The model under review builds one solid part; all positions refer to its coordinate system, in mm. Face numbers are marked on the shaded views. Round coordinates to 2 decimals unless told otherwise and drop trailing zeros. Order: outer loops, then holes, each group sorted by start corner. A loop starts at its lowest first (then second) coordinate and runs counter-clockwise, first axis right, second up. Notation, with made-up numbers: M 2,7.5 L 56,7.5 A21 ccw 56,27.5 Z; hole C 76,-13.75 d10. An arc over 180 degrees is marked long. Use a Markdown table: item, result. Add a question column.
1. To check wall thickness, follow probe 1 along Y at (x, z) = (0, 87.5); probe 2 along Y at (x, z) = (0, -47); probe 3 along Z at (x, y) = (8.5, -10). State the ranges of each line that lie inside material, in increasing order.
2. Insertion check: P1, Ø15, axis at x = -1, y = -2, coming from the -Z side; P2, Ø2, axis at y = 8, z = 72.5, coming from the +X side; P3, Ø5, axis at x = 8.5, y = 4.5, coming from the -Z side; P4, Ø8, axis at y = 10, z = -82.5, coming from the +X side. Each pin has a flat end and moves straight along its axis. Give the tip position at first contact, or say it passes through.
3. Consider section A-A on x = 0. State the section outline as (y, z) points, then the cut area to 3 significant figures.
4. Consider section C-C on z = 39.5. State the section outline as (x, y) points.
5. The part is to be moulded in two halves that separate along X. For the marked faces 1, 2 and 3, say which applies: +X half, -X half, draft (parallel to the pull), parting line (faces both ways), or undercut.
from build123d import *

# Parameters (mm, degrees)
FILLET1_R = 2


with BuildPart() as part:
    # Sketch1 → Revolve1 (revolve)
    with BuildSketch(Plane.YZ, mode=Mode.PRIVATE) as revolve1_sk:
        Polygon((10, 115), (19, 115), (19, -115), (15, -115), (15, 75), (10, 75), align=None)
    revolve(revolve1_sk.sketch.rotate(Axis((0, 0, 319.317365216), (0, 0, -1)), 90), axis=Axis((0, 0, 319.317365216), (0, 0, -1)))

    # Fillet1
    fillet1_edges = [part.edges().sort_by_distance(p)[0] for p in [
        (-19, 0, 115),
    ]]
    fillet(fillet1_edges, radius=FILLET1_R)


solid = part.part
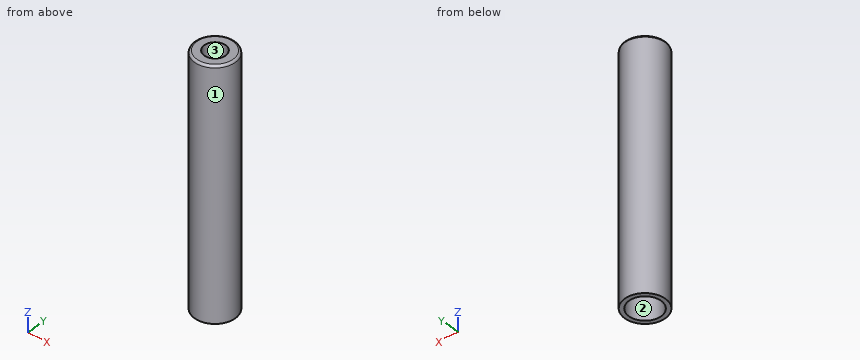
Answer block:
| question | item | result |
|---|---|---|
| 1 | probe 1 | -19 to -10, 10 to 19 |
| 1 | probe 2 | -19 to -15, 15 to 19 |
| 1 | probe 3 | 75 to 115 |
| 2 | P1 | through |
| 2 | P2 | x = 17.66 |
| 2 | P3 | z = 75 |
| 2 | P4 | x = 18.03 |
| 3 | outline | M -19,-115 L -15,-115 L -15,75 L -10,75 L -10,115 L -17,115 A2 ccw -19,113 Z; M 10,75 L 15,75 L 15,-115 L 19,-115 L 19,113 A2 ccw 17,115 L 10,115 Z |
| 3 | area | 2,240 mm^2 |
| 4 | outline | C 0,0 d38; hole C 0,0 d30 |
| 5 | face 1 | parting line |
| 5 | face 2 | undercut |
| 5 | face 3 | undercut |
